Design review of the part built by this model. Coordinates are the model's own, in mm. Face numbers are marked on the shaded views. A direction names the side the tool comes from. Give positions to 0.01 mm unless a question says otherwise; leave off trailing zeros. Write each loop counter-clockwise with the first axis right and the second up, starting at its lowest first coordinate (ties: lowest second). Pieces come first, ordered by that corner, then holes. Notation, with made-up numbers: M 20.5,-20 L 29.5,-20 A22 cw 29.5,11 Z; hole C 75,-26 d6. An arc over 180 degrees is marked long. One line per item, written item: value. Start each with the question number.
```python
from build123d import *

# Parameters (mm, degrees)
F0_R     = 10
F1_DEPTH = 25
F3_DEPTH = 100
F4_W     = 70
F4_H     = 15
F5_DEPTH = 20
F6_R     = 7.5
F7_DEPTH = 10


with BuildPart() as f1:
    # F0 (on Right) → F1 (new body)
    with BuildSketch(Plane.YZ):
        with BuildLine():
            Line((0, 70), (0, 0))
            Line((0, 0), (50, 0))
            Line((50, 0), (50, 70))
            ThreePointArc((50, 70), (42.67767, 87.67767), (25, 95))
            ThreePointArc((25, 95), (7.32233, 87.67767), (0, 70))
        make_face()
        with Locations((25, 70)):
            Circle(F0_R, mode=Mode.SUBTRACT)
    extrude(amount=F1_DEPTH)

    # F2 (on face) → F3 (join)
    with BuildSketch(Plane.YZ.offset(25)):
        Polygon((0, 45), (0, 0), (50, 0), (50, 10), (20, 10), (20, 45), align=None)
    extrude(amount=F3_DEPTH)

    # F4 (on face) → F5 (cut)
    with BuildSketch(Plane(origin=(0, 20, 0), x_dir=(-1, 0, 0), z_dir=(0, 1, 0))):
        with Locations((-74, 27.5)):
            Rectangle(F4_W, F4_H)
    extrude(amount=-F5_DEPTH, mode=Mode.SUBTRACT)

    # F6 (on face) → F7 (cut)
    with BuildSketch(Plane.XY.offset(10)):
        with Locations((100, 35)):
            Circle(F6_R)
        with Locations((50, 35)):
            Circle(F6_R)
    extrude(amount=-F7_DEPTH, mode=Mode.SUBTRACT)


solid = f1.part
```
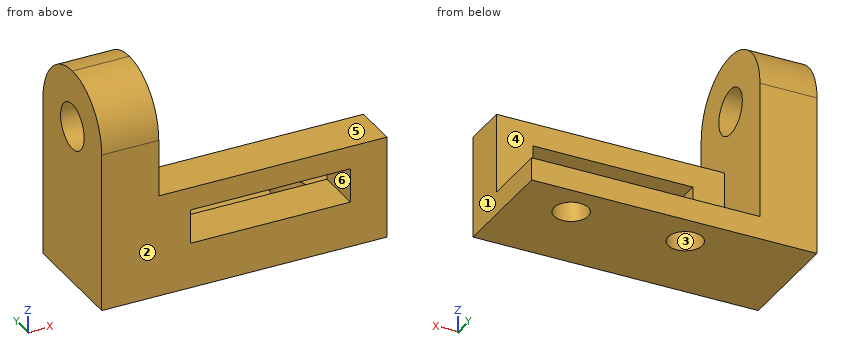
Q1. Take a section at D-D, the plane y = 10. Give the boundary of the cut face in (x, z), then the cut area to 3 significant figures.
Q2. Take a section at C-C, the plane z = 78. Give the boundary of the cut face in (x, y).
Q3. Machinability: for the marked faces 4, 5 and 6, which of the approach directions +Z, -Z, +X, -X, +Y, -Y give a long, thin tool a straight path to every point of the face, cutting with its end or side? Answer none if there is none.
Q4. Take a section at B-B, the plane x = 77. Give the boundary of the cut face in (y, z), then the cut area to 3 significant figures.
Q5. Take a section at A-A, the plane x = 50. Give the boundary of the cut face in (y, z), then the cut area to 3 significant figures.
Q6. The part is to be moulded in two halves that separate along Y. For the marked faces 1, 2 and 3, say which applies: pulls with the +Y half, pulls with the -Y half, needs draft (parallel to the pull), parting line crosses it, or undercut.
Q7. Wall thickness on line 1 (Z direction, x = 85.5, y = 13); line 2 (Y direction, x = 50, z = 3); line 3 (Z direction, x = 9, y = 25): over which ranges is each line inside the solid? List them lowest first. Write a range as from..to.
Q8. For P1, Ø12, axis at y = 13.5, z = 79, coming from the +X side; P2, Ø22, axis at x = 82, y = 6, coming from the +Z side; P3, Ø17.5, axis at x = 89.5, z = 32.5, coming from the +Y side, all flat-tipped, find the tip position at first contact; note any pin that passes through.
Results list:
1. outline: M 0,0 L 125,0 L 125,45 L 25,45 L 25,90 L 0,90 Z; hole M 39,20 L 109,20 L 109,35 L 39,35 Z
1. area: 5,700 mm^2
2. outline: M 0,1.31 L 25,1.31 L 25,19 L 0,19 Z; M 0,31 L 25,31 L 25,48.69 L 0,48.69 Z
3. face 4: +Z, +X, +Y
3. face 5: +Z, +X, +Y, -Y
3. face 6: +Y, -Y
4. outline: M 0,0 L 50,0 L 50,10 L 20,10 L 20,20 L 0,20 Z; M 0,35 L 20,35 L 20,45 L 0,45 Z
4. area: 900 mm^2
5. outline: M 0,0 L 27.5,0 L 27.5,10 L 20,10 L 20,20 L 0,20 Z; M 0,35 L 20,35 L 20,45 L 0,45 Z; M 42.5,0 L 50,0 L 50,10 L 42.5,10 Z
5. area: 750 mm^2
6. face 1: needs draft
6. face 2: pulls with the -Y half
6. face 3: undercut
7. line 1: z = 0..20, 35..45
7. line 2: y = 0..27.5, 42.5..50
7. line 3: z = 0..60, 80..95
8. P1: stops at x = 25
8. P2: stops at z = 45
8. P3: stops at y = 20
